The listing builds one solid part. Answer for the finished solid, in the listing's coordinates (mm). A direction names the side the tool comes from. Give positions to 0.01 mm unless a question says otherwise; leave off trailing zeros. Order: outer loops, then holes, each group sorted by start corner. A loop starts at its lowest first (then second) coordinate and runs counter-clockwise, first axis right, second up. Notation, with made-up numbers: (80, 27) - (86, 27) arc R14 cw to (86, 43) - close; hole circle Ø10 at (77.25, -25.5). An arc over 180 degrees is marked (long way). Answer in a Markdown table with one row per item. Add a question column.
```python
from build123d import *

# Parameters (mm, degrees)
SKETCHSIDE_R                    = 0.5
BOSSEXTRUDESIDE_DEPTH           = 22
CUTEXTRUDEDISTALROOM_DEPTH      = 60.939469467
CUTEXTRUDEDISTALROOM_DEPTH_BACK = 60.939469467
SKETCHSESORROOM_W               = 5
SKETCHSESORROOM_H               = 10
CUTEXTRUDESENSORROOM_DEPTH      = 10
CUTEXTRUDESTRONGSIDE_DEPTH      = 60.939469467
CUTEXTRUDESTRONGSIDE_DEPTH_BACK = 60.939469467
SKETCHSTRONGSIDE_W              = 30
SKETCHSTRONGSIDE_H              = 4
FILLETSTRONGSIDE_R              = 50
FILLETSIDE_R                    = 2
CUTEXTRUDESPRINGROOM_DEPTH      = 60.939469467
CUTEXTRUDESPRINGROOM_DEPTH_BACK = 60.939469467
SKETCHSPRINGROOM_W              = 6
SKETCHSPRINGROOM_H              = 7


with BuildPart() as part:
    # SketchSide → BossExtrudeSide (new body)
    with BuildSketch(Plane(origin=(0, 0, 0), x_dir=(1, 0, 0), z_dir=(0, 1, 0))):
        with BuildLine():
            Line((-2.5, -24.778081045), (-2.5, 0))
            ThreePointArc((-2.5, 0), (0, 2.5), (2.5, 0))
            Line((2.5, 0), (2.5, -53.2))
            ThreePointArc((2.5, -53.2), (0, -55.7), (-2.5, -53.2))
            Line((-2.5, -53.2), (-2.5, -24.778081045))
        make_face()
        with Locations(Location((0, 0, 0), (0, 0, 270))):
            Circle(SKETCHSIDE_R, mode=Mode.SUBTRACT)
        with Locations(Location((0, -53.2, 0), (0, 0, 270))):
            Circle(SKETCHSIDE_R, mode=Mode.SUBTRACT)
    extrude(amount=BOSSEXTRUDESIDE_DEPTH)

    # SketchDistalRoom → CutExtrudeDistalRoom (cut, two sides: drawn at the far end of the back side and taken through both)
    with BuildSketch(Plane(origin=(0, 0, 0), x_dir=(0, 0, -1), z_dir=(1, 0, 0)).offset(-CUTEXTRUDEDISTALROOM_DEPTH_BACK)):
        Polygon((-44.7, 13.5), (-47.7, 13.5), (-47.7, 17.5), (-55.7, 17.5), (-55.7, 4.5), (-44.7, 4.5), align=None)
    extrude(amount=CUTEXTRUDEDISTALROOM_DEPTH + CUTEXTRUDEDISTALROOM_DEPTH_BACK, mode=Mode.SUBTRACT)

    # SketchSesorRoom → CutExtrudeSensorRoom (cut)
    with BuildSketch(Plane(origin=(0, 0, 0), x_dir=(0, 0, -1), z_dir=(1, 0, 0))):
        with Locations((-34.2, 9)):
            Rectangle(SKETCHSESORROOM_W, SKETCHSESORROOM_H)
    extrude(amount=-CUTEXTRUDESENSORROOM_DEPTH, mode=Mode.SUBTRACT)

    # SketchStrongSide → CutExtrudeStrongSide (cut, two sides: drawn at the far end of the back side and taken through both)
    with BuildSketch(Plane(origin=(0, 0, 0), x_dir=(0, 0, -1), z_dir=(1, 0, 0)).offset(-CUTEXTRUDESTRONGSIDE_DEPTH_BACK)):
        with Locations((-12.5, 20)):
            Rectangle(SKETCHSTRONGSIDE_W, SKETCHSTRONGSIDE_H)
    extrude(amount=CUTEXTRUDESTRONGSIDE_DEPTH + CUTEXTRUDESTRONGSIDE_DEPTH_BACK, mode=Mode.SUBTRACT)

    # FilletStrongSide
    # the kernel refuses this fillet: 50 mm, written as the material it adds along each edge
    with BuildSketch(Plane(origin=(2.5, 18, 27.5), x_dir=(0, 1, 0), z_dir=(-1, 0, 0))) as filletstrongside_piece_1:
        with BuildLine():
            CenterArc((50, 19.595917942), FILLETSTRONGSIDE_R, 180, 23.073918066)
            Line((0, 19.595917942), (-1, 19.595917942))
            Line((-1, 19.595917942), (-1, 0))
            Line((-1, 0), (0, -1))
            ThreePointArc((0, -1), (2, -1), (3.08, -0.391918359))
            Line((3.08, -0.391918359), (4, 0))
        make_face()
    extrude(amount=5)

    # FilletSide
    filletside_edges = [part.edges().sort_by_distance(p)[0] for p in [
        (0, 22, 27.5),
    ]]
    fillet(filletside_edges, radius=FILLETSIDE_R)

    # SketchSpringRoom → CutExtrudeSpringRoom (cut, two sides: drawn at the far end of the back side and taken through both)
    with BuildSketch(Plane(origin=(0, 0, 0), x_dir=(0, 0, -1), z_dir=(1, 0, 0)).offset(-CUTEXTRUDESPRINGROOM_DEPTH_BACK)):
        with Locations((-0.5, 9)):
            Rectangle(SKETCHSPRINGROOM_W, SKETCHSPRINGROOM_H)
    extrude(amount=CUTEXTRUDESPRINGROOM_DEPTH + CUTEXTRUDESPRINGROOM_DEPTH_BACK, mode=Mode.SUBTRACT)


solid = part.part
```
(1) Find section B-B, the plane y = 7.5. Write down the section's boundary in (x, z).
(2) Find section C-C, the plane x = -1.85. Write down the section's boundary in (y, z).
(3) Each of these flat-tipped pins is pushed along its axis until it touches: P1, Ø2.5, axis at x = 0.5, z = 0.5, coming from the +Y side; P2, Ø1.5, axis at x = 1, y = 11.5, coming from the +Z side; P3, Ø1.2, axis at x = -1, y = 16.5, coming from the +Z side. Where does it stop, or does it pass through?
(4) For faces 5 (the face through (-2.5, 11, 26)), 6 (the face through (0, 5.5, 1)), 7 (the face through (-1, 9, 31.7)), 8 (the face through (0, 13.5, 46)), determine the directions among +Z, -Z, +X, -X, +Y, -Y from which every point of the face is accessible in a straight line to the end or side of a thin tool.
(5) Find section A-A, the plane z = 50. Write down the section's boundary in (x, y), plus the area to 3 significant figures.
(6) Find section D-D, the plane y = 16.25. Write down the section's boundary in (x, z), plus the area to 3 significant figures.
(7) Straight lines are drawn through the part: line 1 (Z direction, x = 0, y = 2.45); line 2 (Z direction, x = 0, y = 16.45); line 3 (Z direction, x = -2.1, y = 12). For each, find the intervals that lie inside material, in ascending order.
(8) The mould has two halves that part along Z. Classify faces 1 (the face through (-0.488, 2.712, -0.108)), 2 (the face through (0, 19.7, 52.7)), 3 (the face through (0, 15, 47.7)), 4 (the face through (0, 18, 3)): +Z half, -Z half, draft (parallel to the pull), parting line (faces both ways), or undercut.
Answer key:
| question | item | result |
|---|---|---|
| 1 | outline | (-2.5, 3.5) - (2.5, 3.5) - (2.5, 44.7) - (-2.5, 44.7) - (-2.5, 36.7) - (0, 36.7) - (0, 31.7) - (-2.5, 31.7) - close |
| 2 | outline | (0, -1.68) - (5.5, -1.68) - (5.5, 3.5) - (12.5, 3.5) - (12.5, -1.68) - (18, -1.68) - (18, 7.9) arc R50 cw to (21.85, 27.13) arc R2 ccw to (22, 27.9) - (22, 54.88) - (17.5, 54.88) - (17.5, 47.7) - (13.5, 47.7) - (13.5, 44.7) - (4.5, 44.7) - (4.5, 54.88) - (0, 54.88) - close; hole (4, 31.7) - (14, 31.7) - (14, 36.7) - (4, 36.7) - close |
| 3 | P1 | y = 18 |
| 3 | P2 | z = 44.7 |
| 3 | P3 | z = 47.7 |
| 4 | face 5 | +Z, -Z, -X, +Y, -Y |
| 4 | face 6 | -Z, +X, -X |
| 4 | face 7 | -X |
| 4 | face 8 | +Z, +X, -X |
| 5 | outline | (-2.5, 0) - (2.5, 0) - (2.5, 4.5) - (-2.5, 4.5) - close; (-2.5, 17.5) - (2.5, 17.5) - (2.5, 22) - (-2.5, 22) - close |
| 5 | area | 45.0 mm² |
| 6 | outline | (-2.5, 0) arc R2.5 ccw to (2.5, 0) - (2.5, 47.7) - (-2.5, 47.7) - close; hole circle Ø1 at (0, 0) |
| 6 | area | 248 mm² |
| 7 | line 1 | -2.5 to -0.5, 0.5 to 52.7, 53.7 to 55.7 |
| 7 | line 2 | -2.5 to -0.5, 0.5 to 47.7 |
| 7 | line 3 | 3.5 to 31.7, 36.7 to 44.7 |
| 8 | face 1 | undercut |
| 8 | face 2 | undercut |
| 8 | face 3 | +Z half |
| 8 | face 4 | draft |
